For this review, take the finished solid that the model builds, in its own axes (mm). A direction names the side the tool comes from. Coordinates: 2 decimals unless noted, no trailing zeros. Write each loop counter-clockwise with the first axis right and the second up, starting at its lowest first coordinate (ties: lowest second). Pieces come first, ordered by that corner, then holes. Notation, with made-up numbers: M 37,-31.5 L 88,-31.5 A12 cw 88,-14.5 Z; hole C 70.5,55 d11. An arc over 180 degrees is marked long. One line per question, with ' | ' between items.
from build123d import *

# Parameters (mm, degrees)
SKETCH2_R           = 1.905
BOSS_EXTRUDE1_DEPTH = 13.97
SKETCH7_W           = 8.89
SKETCH7_H           = 13.736668288
CUT_EXTRUDE1_DEPTH  = 8.89
SKETCH8_W           = 15.99010018
SKETCH8_H           = 8.89
CUT_EXTRUDE2_DEPTH  = 38.354
CUT_EXTRUDE4_START  = -2.54
CUT_EXTRUDE4_DEPTH  = 8.89
FILLET1_R           = 5.08
CHAMFER1_SIZE       = 2.38
CHAMFER1_SIZE_2     = 1.683044883
CUT_EXTRUDE5_DEPTH  = 8.89


with BuildPart() as part:
    # Sketch2 → Boss-Extrude1 (new body)
    with BuildSketch(Plane.XY):
        with BuildLine():
            Line((-63.967060474, -130.859635454), (-76.667060474, -130.859635454))
            Line((-76.667060474, -130.859635454), (-92.67813479, -72.364175631))
            Line((-92.67813479, -72.364175631), (-93.509383851, -33.790725064))
            Line((-93.509383851, -33.790725064), (-83.152945307, -43.960741607))
            Line((-83.152945307, -43.960741607), (-82.481678491, -58.768900565))
            ThreePointArc((-82.481678491, -58.768900565), (-74.536997263, -66.480585097), (-63.5, -67.359635454))
            ThreePointArc((-63.5, -67.359635454), (-67.758675084, -97.020798424), (-63.967060474, -126.745275894))
            Line((-63.967060474, -126.745275894), (-63.967060474, -130.859635454))
        make_face()
        with Locations((-88.424072453, -48.053785371)):
            Circle(SKETCH2_R, mode=Mode.SUBTRACT)
        with Locations((-76.667060474, -71.37070905)):
            Circle(SKETCH2_R, mode=Mode.SUBTRACT)
    extrude(amount=-BOSS_EXTRUDE1_DEPTH)

    # Sketch7 → Cut-Extrude1 (cut)
    with BuildSketch(Plane(origin=(-84.97111807, -3.851815205, 0), x_dir=(0, 0, -1), z_dir=(0.9989741366022207, 0.04528437257871392, 0))):
        with Locations((6.985, -54.652422544)):
            Rectangle(SKETCH7_W, SKETCH7_H)
    extrude(amount=-CUT_EXTRUDE1_DEPTH, mode=Mode.SUBTRACT)

    # Sketch8 → Cut-Extrude2 (cut)
    with BuildSketch(Plane(origin=(2.163872462, -47.735068453, 0), x_dir=(0.9989741366022207, 0.04528437257871392, 0), z_dir=(0.04528437257871392, -0.9989741366022207, 0))):
        with Locations((-85.953326255, -6.985)):
            Rectangle(SKETCH8_W, SKETCH8_H)
    extrude(amount=-CUT_EXTRUDE2_DEPTH, mode=Mode.SUBTRACT)

    # Sketch9 → Cut-Extrude4 (cut)
    with BuildSketch(Plane.XY.offset(CUT_EXTRUDE4_START)):
        with BuildLine():
            Line((-82.481678491, -58.768900565), (-84.301115942, -65.397976437))
            ThreePointArc((-84.301115942, -65.397976437), (-80.869859076, -76.151152323), (-71.419742843, -82.323641162))
            Line((-71.419742843, -82.323641162), (-53.044010763, -68.759286996))
            Line((-53.044010763, -68.759286996), (-82.481678491, -58.768900565))
        make_face()
    extrude(amount=-CUT_EXTRUDE4_DEPTH, mode=Mode.SUBTRACT)

    # Fillet1
    fillet1_edges = [part.edges().sort_by_distance(p)[0] for p in [
        (-76.667060474, -130.859635454, -6.985),
    ]]
    fillet(fillet1_edges, radius=FILLET1_R)

    # Chamfer1
    # the kernel refuses this chamfer: 2.38, 1.683044883 mm, written as the material it takes off along each edge
    with BuildSketch(Plane(origin=(-93.509383851, -33.790725064, 6.120605511), x_dir=(-0.005952870242771505, -0.9999822815109639, 0), z_dir=(0, 0, -1))) as chamfer1_piece_1:
        Polygon((CHAMFER1_SIZE * 0.999621916911, -CHAMFER1_SIZE * 0.0274958766106), (CHAMFER1_SIZE_2 * 0.69639613284, -CHAMFER1_SIZE_2 * 0.717657596567), (0, 0), align=None)
    extrude(amount=26.211211023, mode=Mode.SUBTRACT)

    # Sketch10 → Cut-Extrude5 (cut)
    with BuildSketch(Plane.XY.offset(-11.43)):
        with BuildLine():
            add(Edge.make_bspline(
                [(-91.586396319, -42.98933193), (-93.184858066, -42.868299271), (-96.695097172, -48.735009259), (-91.017537843, -56.721704987), (-87.675016869, -48.216390701), (-90.229073725, -43.092105964), (-91.586396319, -42.98933193)],
                knots=[0, 0, 0, 0, 0.267383985, 0.513635097, 0.772952762, 1, 1, 1, 1], degree=3))
        make_face()
    extrude(amount=CUT_EXTRUDE5_DEPTH, mode=Mode.SUBTRACT)


solid = part.part
1. Take a section at C-C on y = -56. State the section outline as (x, z) points.
Computed values:
outline: M -93.03,-13.97 L -82.61,-13.97 L -82.61,-11.43 L -91.51,-11.43 L -91.51,-2.54 L -82.61,-2.54 L -82.61,0 L -93.03,0 Z
2. For line 1 along Z through (x, y) = (-90, -42.5); line 2 along X through (y, z) = (-47, -11.5); line 3 along X through (y, z) = (-53.5, -7.25), list the stretches that pass through material, from the lowest coordinate up.
Computed values:
line 1: z = -13.97 to -11.43, -2.54 to 0 | line 2: x = -93.22 to -90.01, -86.84 to -83.02 | line 3: x = -93.08 to -92.67
3. Clearance check with flat-ended pins moving along their axes: P1, Ø3, axis at y = -63.5, z = -10.5, coming from the +X side; P2, Ø8, axis at y = -46.5, z = -9, coming from the -X side; P3, Ø1.5, axis at x = -79.5, z = -5, coming from the +Y side. State where each tip first meets the part, or that it passes through.
Computed values:
P1: stops at x = -77.59 | P2: stops at x = -93.32 | P3: stops at y = -76.92
4. Machinability: for faces 1 (the flat face through (-82.822, -51.261, -12.682)), 2 (the flat face through (-92.27, -39.14, -7.05)), 3 (the flat face through (-68.765, -80.364, -6.923)), 4 (the flat face through (-63.967, -129, -7)), which of the approach directions +Z, -Z, +X, -X, +Y, -Y give a long, thin tool a straight path to every point of the face, cutting with its end or side? Answer none if there is none.
Computed values:
face 1: +Z, -Z, +X, +Y | face 2: +X, +Y | face 3: +Y | face 4: +Z, -Z, +X, -Y
5. Take a section at D-D on x = -81.5. State the section outline as (y, z) points, plus the area to 3 significant figures.
Computed values:
outline: M -113.2,-13.97 L -60.5,-13.97 L -60.5,-11.43 L -75.27,-11.43 L -75.27,-2.54 L -60.5,-2.54 L -60.5,0 L -113.2,0 Z | area: 605 mm2
6. Take a section at A-A on x = -88.25. State the section outline as (y, z) points.
Computed values:
outline: M -88.54,-13.97 L -49.95,-13.97 L -49.95,-11.43 L -65.58,-11.43 L -65.58,-2.54 L -49.95,-2.54 L -49.95,0 L -88.54,0 Z; M -46.16,-13.97 L -38.96,-13.97 L -38.96,-11.43 L -46.16,-11.43 Z; M -46.16,-2.54 L -38.96,-2.54 L -38.96,0 L -46.16,0 Z
7. Draft analysis for pull direction Y (two halves, no side actions). For faces 5 (the flat face through (-85.08, -100.13, -6.89)), 6 (the cylindrical face through (-86.664, -48.783, -12.682)), 7 (the flat face through (-87.8, -39.4, -12.7)), state which applies: pulls with the +Y half, pulls with the -Y half, needs draft (parallel to the pull), parting line crosses it, or undercut.
Computed values:
face 5: pulls with the -Y half | face 6: undercut | face 7: pulls with the +Y half
8. Take a section at B-B on z = -12.25. State the section outline as (x, y) points (1 decimal).
Computed values:
outline: M -93.5,-36.2 L -92.7,-72.4 L -77.7,-127.1 A5.1 ccw -72.8,-130.9 L -64,-130.9 L -64,-126.7 A111.5 cw -63.5,-67.4 A16.3 cw -82.5,-58.8 L -83.2,-44 L -92.3,-35 Z; hole C -88.4,-48.1 d3.8; hole C -76.7,-71.4 d3.8
